Can you work these out from the model? Positions are in its coordinate system, mm. A direction names the side the tool comes from. Give positions to 0.01 mm unless a question says otherwise; leave off trailing zeros. Order: outer loops, then holes, each group sorted by start corner. A loop starts at its lowest first (then second) coordinate and runs counter-clockwise, first axis right, second up. Notation, with made-up numbers: (43, -12) -> (92, -12) arc R18 cw to (92, 23) -> close; hole circle Ø1 at (59.5, 30). An arc over 180 degrees is marked (long way). Answer as a JSON object with one key per item and string values.
```python
from build123d import *

# Parameters (mm, degrees)
RESSALTO_EXTRUS_O1_DEPTH = 3
FILETE1_R                = 1


with BuildPart() as part:
    # Esboço1 → Ressalto-extrusão1 (new body)
    with BuildSketch(Plane.XY):
        Polygon((-8.50739043, 33.509840055), (-43.485746942, 33.509840055), (-43.485746942, -33.566083295), (43.608248957, -33.566083295), (43.608248957, 33.509840055), (15.716409294, 33.509840055), (15.716409294, 4.953578222), (-8.50739043, 4.953578222), align=None)
    extrude(amount=RESSALTO_EXTRUS_O1_DEPTH)

    # Filete1
    filete1_edges = [part.edges().sort_by_distance(p)[0] for p in [
        (43.608248957, -33.566083295, 1.5),
        (-43.485746942, -33.566083295, 1.5),
        (-43.485746942, 33.509840055, 1.5),
        (-8.50739043, 33.509840055, 1.5),
        (-8.50739043, 4.953578222, 1.5),
        (15.716409294, 4.953578222, 1.5),
        (15.716409294, 33.509840055, 1.5),
        (43.608248957, 33.509840055, 1.5),
    ]]
    fillet(filete1_edges, radius=FILETE1_R)


solid = part.part
```
1. If we section it at B-B on z = 2.3: Please give me the cut outline in (x, y).
Worked answers:
{"outline": "(-43.49, -32.57) arc R1 ccw to (-42.49, -33.57) -> (42.61, -33.57) arc R1 ccw to (43.61, -32.57) -> (43.61, 32.51) arc R1 ccw to (42.61, 33.51) -> (16.72, 33.51) arc R1 ccw to (15.72, 32.51) -> (15.72, 5.95) arc R1 cw to (14.72, 4.95) -> (-7.51, 4.95) arc R1 cw to (-8.51, 5.95) -> (-8.51, 32.51) arc R1 ccw to (-9.51, 33.51) -> (-42.49, 33.51) arc R1 ccw to (-43.49, 32.51) -> close"}
2. For faces 1 (the face through (-26, 33.51, 1)), 2 (the face through (15.716, 19, 1)), which set-ups out of +Z, -Z, +X, -X, +Y, -Y let a thin tool reach every point of the face, with its end or its side?
Worked answers:
{"face 1": "+Z, -Z, +X, -X, +Y", "face 2": "+Z, -Z, +Y"}
3. If we section it at A-A on y = 29.5: Please give me the cut outline in (x, z).
Worked answers:
{"outline": "(-43.49, 0) -> (-8.51, 0) -> (-8.51, 3) -> (-43.49, 3) -> close; (15.72, 0) -> (43.61, 0) -> (43.61, 3) -> (15.72, 3) -> close"}
4. Please list where these lines run through material, in increasing order: L1, parallel to X at y = 6.5, z = 2.3; L2, parallel to Y at x = 3.5, z = 1.5.
Worked answers:
{"L1": "-43.49 to -8.51, 15.72 to 43.61", "L2": "-33.57 to 4.95"}
5. If we mould it in two halves opening along X, with no side actions, what happens to faces 3 (the face through (-8.507, 19, 1)), 4 (the face through (-1, -33.566, 1)), 5 (the face through (-43.486, 0, 1))? For each: +X half, -X half, draft (parallel to the pull), parting line (faces both ways), or undercut.
Worked answers:
{"face 3": "undercut", "face 4": "draft", "face 5": "-X half"}
